```python
from build123d import *

# Parameters (mm, degrees)
BOSS_EXTRUDE1_DEPTH                             = 12.7
CSK_FOR_M4_FLAT_HEAD_MACHINE_SCREW1_D           = 4.3
CSK_FOR_M4_FLAT_HEAD_MACHINE_SCREW1_CSINK_D     = 9.4
CSK_FOR_M4_FLAT_HEAD_MACHINE_SCREW1_CSINK_ANGLE = 90
CHAMFER1_SIZE                                   = 16
SKETCH6_W                                       = 10
SKETCH6_H                                       = 6
BOSS_EXTRUDE2_DEPTH                             = 12.7
FILLET5_R                                       = 8
M3X0_5_TAPPED_HOLE1_D                           = 2.5
FILLET6_START                                   = -1
FILLET6_DEPTH                                   = 15
SKETCH18_W                                      = 25
SKETCH18_H                                      = 19
BOSS_EXTRUDE4_DEPTH                             = 12.7
FILLET11_R                                      = 15
FILLET12_R                                      = 3
M3X0_5_TAPPED_HOLE2_D                           = 2.5
CSK_FOR_M4_FLAT_HEAD_MACHINE_SCREW2_D           = 4.5
CSK_FOR_M4_FLAT_HEAD_MACHINE_SCREW2_CSINK_D     = 9.9
CSK_FOR_M4_FLAT_HEAD_MACHINE_SCREW2_CSINK_ANGLE = 90


with BuildPart() as part:
    # Sketch1 → Boss-Extrude1 (new body)
    with BuildSketch(Plane(origin=(0, 0, 0), x_dir=(1, 0, 0), z_dir=(0, 1, 0))):
        Polygon((-5, 274), (5, 274), (5, 255), (255, 255), (255, -271), (245, -271), (245, -255), (-245, -255), (-245, -271), (-255, -271), (-255, 255), (-5, 255), align=None)
    extrude(amount=BOSS_EXTRUDE1_DEPTH)

    # CSK for M4 Flat Head Machine Screw1 (through all)
    with Locations(Plane(origin=(0, 12.7, 0), x_dir=(1, 0, 0), z_dir=(0, 1, 0))):
        with Locations((0, 269), (-250, -266), (250, -266)):
            CounterSinkHole(CSK_FOR_M4_FLAT_HEAD_MACHINE_SCREW1_D / 2, CSK_FOR_M4_FLAT_HEAD_MACHINE_SCREW1_CSINK_D / 2, counter_sink_angle=CSK_FOR_M4_FLAT_HEAD_MACHINE_SCREW1_CSINK_ANGLE)

    # Chamfer1
    chamfer1_edges = [part.edges().sort_by_distance(p)[0] for p in [
        (245, 6.35, 255),
        (-245, 6.35, 255),
    ]]
    chamfer(chamfer1_edges, length=CHAMFER1_SIZE - 0.0001)  # a hair under: the kernel refuses the full size

    # Sketch6 → Boss-Extrude2 (add)
    with BuildSketch(Plane(origin=(0, 12.7, 0), x_dir=(1, 0, 0), z_dir=(0, 1, 0))):
        with Locations((-250, 258)):
            Rectangle(SKETCH6_W, SKETCH6_H)
        with Locations((250, 258)):
            Rectangle(SKETCH6_W, SKETCH6_H)
    extrude(amount=-BOSS_EXTRUDE2_DEPTH)

    # Fillet5
    # the kernel refuses this fillet: 8 mm, written as the material it adds along each edge
    with BuildSketch(Plane(origin=(245, 12.7, -255), x_dir=(0, 0, -1), z_dir=(0, -1, 0))) as fillet5_piece_1:
        with BuildLine():
            CenterArc((8, -7.745966692), FILLET5_R, 104.477512186, 75.522487814)
            Line((0, -7.745966692), (-0.16, -7.745966692))
            Line((-0.16, -7.745966692), (-0.16, 0))
            Line((-0.16, 0), (0, 0.16))
            ThreePointArc((0, 0.16), (3, 0.16), (5.96, 0.154919334))
            Line((5.96, 0.154919334), (6, 0))
        make_face()
    extrude(amount=12.7)
    with BuildSketch(Plane(origin=(-245, 12.7, -255), x_dir=(1, 0, 0), z_dir=(0, -1, 0))) as fillet5_piece_2:
        with BuildLine():
            CenterArc((7.745966692, -8), FILLET5_R, 90, 75.522487814)
            Line((0, -6), (-0.154919334, -5.96))
            ThreePointArc((-0.154919334, -5.96), (-0.16, -3), (-0.16, 0))
            Line((-0.16, 0), (0, 0.16))
            Line((0, 0.16), (7.745966692, 0.16))
            Line((7.745966692, 0.16), (7.745966692, 0))
        make_face()
    extrude(amount=12.7)

    # M3x0.5 Tapped Hole1 (through all)
    with Locations(Plane(origin=(0, 12.7, 0), x_dir=(1, 0, 0), z_dir=(0, 1, 0))):
        with Locations((-250, 256.5), (250, 256.5), (239.607695155, -260), (-239.607695155, -260), (0, 258)):
            Hole(M3X0_5_TAPPED_HOLE1_D / 2)

    # Fillet6: read off the stored shape, not the designer's step
    # Fillet6 outline → Fillet6 (cut)
    with BuildSketch(Plane(origin=(0, 0, 0), x_dir=(1, 0, 0), z_dir=(0, 1, 0)).offset(FILLET6_START)):
        with BuildLine():
            ThreePointArc((255, -266), (253.535533906, -269.535533906), (250, -271))
            Line((250, -271), (255, -271))
            Line((255, -271), (255, -266))
        make_face()
        with BuildLine():
            ThreePointArc((247.071067812, -271), (245.15765065, -270.619397663), (243.535533906, -269.535533906))
            Line((243.535533906, -269.535533906), (245, -271))
            Line((245, -271), (247.071067812, -271))
        make_face()
        with BuildLine():
            ThreePointArc((-243.535533906, -269.535533906), (-245.15765065, -270.619397663), (-247.071067812, -271))
            Line((-247.071067812, -271), (-245, -271))
            Line((-245, -271), (-243.535533906, -269.535533906))
        make_face()
        with BuildLine():
            Line((-255, -271), (-250, -271))
            ThreePointArc((-250, -271), (-253.535533906, -269.535533906), (-255, -266))
            Line((-255, -266), (-255, -271))
        make_face()
    extrude(amount=FILLET6_DEPTH, mode=Mode.SUBTRACT)

    # Sketch18 → Boss-Extrude4 (add)
    with BuildSketch(Plane.XZ):
        with Locations((17.5, -264.5)):
            Rectangle(SKETCH18_W, SKETCH18_H)
        with Locations((-17.5, -264.5)):
            Rectangle(SKETCH18_W, SKETCH18_H)
    extrude(amount=-BOSS_EXTRUDE4_DEPTH)

    # Fillet11
    fillet11_edges = [part.edges().sort_by_distance(p)[0] for p in [
        (30, 6.35, -255),
        (-30, 6.35, -255),
        (-229.0001, 6.35, 255),
        (229.0001, 6.35, 255),
    ]]
    fillet(fillet11_edges, radius=FILLET11_R)

    # Fillet12
    fillet12_edges = [part.edges().sort_by_distance(p)[0] for p in [
        (30, 6.35, -274),
        (-30, 6.35, -274),
        (-245, 6.35, -261),
        (-255, 6.35, -261),
        (245, 6.35, -261),
        (255, 6.35, -261),
    ]]
    fillet(fillet12_edges, radius=FILLET12_R)

    # M3x0.5 Tapped Hole2 (through all)
    with Locations(Plane(origin=(0, 12.7, 0), x_dir=(1, 0, 0), z_dir=(0, 1, 0))):
        with Locations((27, 257), (-27, 271), (-27, 261)):
            Hole(M3X0_5_TAPPED_HOLE2_D / 2)

    # CSK for M4 Flat Head Machine Screw2 (through all)
    with Locations(Plane(origin=(0, 12.7, 0), x_dir=(1, 0, 0), z_dir=(0, 1, 0))):
        with Locations((-210, -217), (-187, -210), (-86, -210), (-210, -116), (-210, -15), (-210, 86), (-210, 187), (-217, 210), (-116, 210), (-15, 210), (86, 210), (187, 210), (210, 217), (210, 116), (210, 15), (210, -86), (210, -187), (217, -210), (116, -210), (15, -210)):
            CounterSinkHole(CSK_FOR_M4_FLAT_HEAD_MACHINE_SCREW2_D / 2, CSK_FOR_M4_FLAT_HEAD_MACHINE_SCREW2_CSINK_D / 2, counter_sink_angle=CSK_FOR_M4_FLAT_HEAD_MACHINE_SCREW2_CSINK_ANGLE)


solid = part.part
```
Geometry: final body of the model. Coordinates: model frame, mm. A direction names the side the tool comes from. Round coordinates to 2 decimals unless told otherwise and drop trailing zeros. Order: outer loops, then holes, each group sorted by start corner. A loop starts at its lowest first (then second) coordinate and runs counter-clockwise, first axis right, second up. Notation, with made-up numbers: (-38, 64) - (-7, 64) arc R14 ccw to (-7, 68) - close; hole circle Ø6 at (76.25, -30.5). An arc over 180 degrees is marked (long way). Write item = value, one per line. Start each with the question number.
Q1. Pull-direction query (X, two-part tool) for faces 1 (the flat face through (-4, 12.7, 2)), 2 (the flat face through (-142, 6, -255)), 3 (the flat face through (-255, 6, 8)); classes: +X half, -X half, draft (parallel to the pull), parting line (faces both ways), or undercut.
Q2. Cut plane A-A on y = 3.5. Give the number of separate pieces and of enclosed holes in the cut face, and give its area (3 significant figures).
Q3. Access query for faces 4 (the flat face through (255, 6, 0)), 5 (the flat face through (3, 6, 255)), 6 (the cylindrical face through (-34.51, 6.44, -259.28)). Directions: +Z, -Z, +X, -X, +Y, -Y. A direction counts if a zero-diameter tool reaches every point of the face in a straight line with its end or side. Return the directions, or none.
Q4. Ray query, line 1 (X direction, y = 6.5, z = -210); line 2 (X direction, y = 3.75, z = 210); line 3 (Z direction, x = -27, y = 3.75). Return the intervals inside material, ascending. Write a range as from..to.
Q5. Cut plane B-B on x = 55.5. Return the cut outline in (y, z).
Q6. Pin query (flat end, axial travel): pin 1 (4 mm diameter, centred on x = 250.5, y = 5, fed in from -Z); pin 2 (6 mm diameter, centred on x = 64, y = 10.5, fed in from +Z); pin 3 (7 mm diameter, centred on x = 86, z = -210, fed in from +Y). Return the tip coordinate at first contact, or that it passes through.
Outcome:
q1.face_1 = draft
q1.face_2 = undercut
q1.face_3 = -X half
q2.separate_pieces = 1
q2.enclosed_holes = 31
q2.area = 262,000 mm^2
q3.face_4 = +Z, -Z, +X, +Y, -Y
q3.face_5 = +Z, +Y, -Y
q3.face_6 = -Z, +Y, -Y
q4.line_1 = -255..-219.25, -214.75..-118.25, -113.75..-17.25, -12.75..83.75, 88.25..184.75, 189.25..255
q4.line_2 = -255..-189.25, -184.75..-88.25, -83.75..12.75, 17.25..113.75, 118.25..214.75, 219.25..255
q4.line_3 = -274..-272.25, -269.75..-262.25, -259.75..255
q5.outline = (0, -255) - (12.7, -255) - (12.7, 255) - (0, 255) - close
q6.pin_1 = -261
q6.pin_2 = 255
q6.pin_3 = 11.25
